from build123d import *

# Parameters (mm, degrees)
SKETCH1_R           = 114.3
BOSS_EXTRUDE1_DEPTH = 12.7
SKETCH2_W           = 12.7
SKETCH2_H           = 76.2
BOSS_EXTRUDE2_DEPTH = 34.798
SKETCH3_W           = 12.7
SKETCH3_H           = 76.2
BOSS_EXTRUDE3_DEPTH = 28.740401289
CUT_EXTRUDE1_START  = -6.35
SKETCH4_W           = 28.393004938
SKETCH4_H           = 63.5
CUT_EXTRUDE1_DEPTH  = 6.35
SKETCH5_W           = 12.954
SKETCH5_H           = 12.954
CUT_EXTRUDE3_DEPTH  = 19.05


with BuildPart() as part:
    # Sketch1 → Boss-Extrude1 (new body)
    with BuildSketch(Plane(origin=(0, 0, 0), x_dir=(1, 0, 0), z_dir=(0, 1, 0))):
        with Locations(Location((-32.882992553, 35.040938939, 0), (0, 0, 270))):
            Circle(SKETCH1_R)
    extrude(amount=BOSS_EXTRUDE1_DEPTH)


with BuildPart() as body_2:
    # Sketch2 → Boss-Extrude2 (new body)
    with BuildSketch(Plane(origin=(-68.183595193, 12.7, 21.019137782), x_dir=(1, 0, 0), z_dir=(0, 1, 0))):
        with Locations((-28.710414214, 81.861212069)):
            Rectangle(SKETCH2_W, SKETCH2_H)
    extrude(amount=-BOSS_EXTRUDE2_DEPTH)


with BuildPart() as body_3:
    # Sketch3 → Boss-Extrude3 (new body)
    with BuildSketch(Plane(origin=(0, 12.7, 4.049059252), x_dir=(1, 0, 0), z_dir=(0, 1, 0))):
        with Locations((35.146495172, 64.834549154)):
            Rectangle(SKETCH3_W, SKETCH3_H)
    extrude(amount=-BOSS_EXTRUDE3_DEPTH)


with BuildPart() as part_1:
    add(part.part)

    # Combine1: cut body 2, body 3
    add(body_2.part, mode=Mode.SUBTRACT)
    add(body_3.part, mode=Mode.SUBTRACT)

    # Sketch4 → Cut-Extrude1 (cut)
    with BuildSketch(Plane(origin=(0, 12.7, 0), x_dir=(1, 0, 0), z_dir=(0, 1, 0)).offset(CUT_EXTRUDE1_START)):
        with BuildLine():
            ThreePointArc((81.417007447, 35.040938939), (78.08126298, 62.45305294), (68.268731087, 88.265170308))
            Line((68.268731087, 88.265170308), (41.496495172, 88.265170308))
            Line((41.496495172, 88.265170308), (41.496495172, 24.765170308))
            Line((41.496495172, 24.765170308), (80.954165612, 24.765170308))
            ThreePointArc((80.954165612, 24.765170308), (81.30123836, 29.897845426), (81.417007447, 35.040938939))
        make_face()
        with BuildLine():
            Line((84.866092825, 88.265170308), (68.268731087, 88.265170308))
            ThreePointArc((68.268731087, 88.265170308), (78.08126298, 62.45305294), (81.417007447, 35.040938939))
            ThreePointArc((81.417007447, 35.040938939), (81.30123836, 29.897845426), (80.954165612, 24.765170308))
            Line((80.954165612, 24.765170308), (84.866092825, 24.765170308))
            Line((84.866092825, 24.765170308), (84.866092825, 88.265170308))
        make_face()
        with Locations((-117.440511876, 60.842074288)):
            Rectangle(SKETCH4_W, SKETCH4_H)
        with BuildLine():
            Line((-131.637014345, 29.092074288), (-131.637014345, 92.592074288))
            ThreePointArc((-131.637014345, 92.592074288), (-143.966610555, 61.96527387), (-147.028080092, 29.092074288))
            Line((-147.028080092, 29.092074288), (-131.637014345, 29.092074288))
        make_face()
        with BuildLine():
            Line((-103.244009407, 29.092074288), (-131.637014345, 29.092074288))
            Line((-131.637014345, 29.092074288), (-147.028080092, 29.092074288))
            ThreePointArc((-147.028080092, 29.092074288), (-146.817975763, 25.913529623), (-146.519377256, 22.742074288))
            Line((-146.519377256, 22.742074288), (-103.244009407, 22.742074288))
            Line((-103.244009407, 22.742074288), (-103.244009407, 29.092074288))
        make_face()
        with BuildLine():
            ThreePointArc((-127.651842399, 98.942074288), (-129.696504455, 95.799756515), (-131.637014345, 92.592074288))
            Line((-131.637014345, 92.592074288), (-103.244009407, 92.592074288))
            Line((-103.244009407, 92.592074288), (-103.244009407, 98.942074288))
            Line((-103.244009407, 98.942074288), (-127.651842399, 98.942074288))
        make_face()
        with BuildLine():
            Line((41.496495172, 22.742074288), (80.75339215, 22.742074288))
            ThreePointArc((80.75339215, 22.742074288), (80.858277027, 23.753175898), (80.954165612, 24.765170308))
            Line((80.954165612, 24.765170308), (41.496495172, 24.765170308))
            Line((41.496495172, 24.765170308), (41.496495172, 22.742074288))
        make_face()
        with BuildLine():
            ThreePointArc((68.268731087, 88.265170308), (65.240150005, 93.661233159), (61.923986686, 98.885489901))
            Line((61.923986686, 98.885489901), (41.496495172, 98.885489901))
            Line((41.496495172, 98.885489901), (41.496495172, 88.265170308))
            Line((41.496495172, 88.265170308), (68.268731087, 88.265170308))
        make_face()
    extrude(amount=CUT_EXTRUDE1_DEPTH, mode=Mode.SUBTRACT)

    # Sketch5 → Cut-Extrude3 (cut)
    with BuildSketch(Plane.XY.offset(79.259061061)):
        with Locations((-64.02495724, 6.223)):
            Rectangle(SKETCH5_W, SKETCH5_H)
        with Locations((-2.04895724, 6.223)):
            Rectangle(SKETCH5_W, SKETCH5_H)
    extrude(amount=-CUT_EXTRUDE3_DEPTH, mode=Mode.SUBTRACT)


solid = part_1.part
Check sheet for the modelled part. Datum: model origin and axes. Units: mm. A direction names the side the tool comes from. Give positions to 0.01 mm unless a question says otherwise; leave off trailing zeros. Loops run counter-clockwise (first coordinate to the right, second up) from the corner with the lowest first, then second, coordinate; pieces in that order, holes last. Notation, with made-up numbers: M 48.25,-26 L 104.25,-26 A26 ccw 104.25,8 Z; hole C -16,27.25 d6. An arc over 180 degrees is marked long. Answer as a JSON object with one key per item and string values. Group by question number.
Q1. Go/stop test with flat-tipped pins: P1, Ø3, axis at x = -42, y = 5, coming from the -Z side; P2, Ø1.9, axis at x = 69, y = 9.5, coming from the -Z side; P3, Ø6.5, axis at y = 3.5, z = 71, coming from the +X side. Record where each tip stops, or that it passes through.
Q2. Cross-section at A-A on z = -55.5. Record the cut outline in (x, y), then the cut area to 3 significant figures.
Q3. Access from +Z, -Z, +X, -X, +Y, -Y to the whole of each face (thin tool, end or side, straight path). Record for faces 1 (the flat face through (-57.548, 6, 69)), 2 (the flat face through (61, 9, -22.742)), 3 (the flat face through (42, 8, -98.885)), 4 (the flat face through (-90.544, 6, -60)).
Q4. Material ranges on line 1 along X through (y, z) = (2, -52); line 2 along X through (y, z) = (6.25, -94.5); line 3 along Z through (x, y) = (-36, 2), recorded low to high. Write a range as [from, to].
Q5. Cross-section at B-B on x = -93.5. Record the cut outline in (y, z).
Q6. Release check for a two-part mould opening along X. For faces 5 (the cylindrical face through (-28.229, 6.261, -149.246)), 6 (the flat face through (4.428, 6, 67)), 7 (the flat face through (61, 6.35, -61)), 8 (the flat face through (41.496, 4, -60)) record: released by +X, released by -X, zero draft, split by the parting line, or undercut.
Q7. Cross-section at D-D on x = 51.5. Record the cut outline in (y, z).
Q8. Cross-section at C-C on y = 3.25. Record the cut outline in (x, z), then the cut area to 3 significant figures.
Evaluation:
{
 "1": {"P1": "stops at z = -149.09", "P2": "stops at z = -22.74", "P3": "stops at x = 17.1"},
 "2": {"outline": "M -145.34,0 L -103.24,0 L -103.24,6.35 L -145.34,6.35 Z; M -90.54,0 L 28.8,0 L 28.8,12.7 L -90.54,12.7 Z; M 41.5,0 L 79.57,0 L 79.57,6.35 L 41.5,6.35 Z", "area": "2,020 mm2"},
 "3": {"face 1": "+Z, +Y, -Y", "face 2": "+X, +Y", "face 3": "+Y", "face 4": "+Y, -Y"},
 "4": {"line 1": "x = [-145.92, -103.24], [-90.54, 28.8], [41.5, 80.15]", "line 2": "x = [-130.5, -103.24], [-90.54, 28.8], [41.5, 64.73]", "line 3": "z = [-149.3, 79.22]"},
 "5": {"outline": "M 0,-131.94 L 12.7,-131.94 L 12.7,-98.94 L 0,-98.94 Z; M 0,-22.74 L 12.7,-22.74 L 12.7,61.86 L 0,61.86 Z"},
 "6": {"face 5": "split by the parting line", "face 6": "undercut", "face 7": "zero draft", "face 8": "undercut"},
 "7": {"outline": "M 0,-112.14 L 12.7,-112.14 L 12.7,-98.89 L 6.35,-98.89 L 6.35,-22.74 L 12.7,-22.74 L 12.7,42.06 L 0,42.06 Z"},
 "8": {"outline": "M -70.5,60.21 L -70.5,72.89 A114.3 ccw long 4.43,73 L 4.43,60.21 L -8.53,60.21 L -8.53,76.63 A114.3 ccw -57.55,76.57 L -57.55,60.21 Z; hole M -103.24,-98.94 L -90.54,-98.94 L -90.54,-22.74 L -103.24,-22.74 Z; hole M 28.8,-98.89 L 41.5,-98.89 L 41.5,-22.69 L 28.8,-22.69 Z", "area": "38,700 mm2"}
}
